Design review of the part built by this model. Coordinates are the model's own, in mm. Face numbers are marked on the shaded views. A direction names the side the tool comes from. Give positions to 0.01 mm unless a question says otherwise; leave off trailing zeros. Write each loop counter-clockwise with the first axis right and the second up, starting at its lowest first coordinate (ties: lowest second). Pieces come first, ordered by that corner, then holes. Notation, with made-up numbers: (83.25, 58.5) -> (107.25, 58.5) arc R30 cw to (107.25, 96.5) -> close; hole circle Ø6 at (-0.5, 8.25). An arc over 180 degrees is marked (long way). Use CSV: the item, a comma, the result in double quotes.
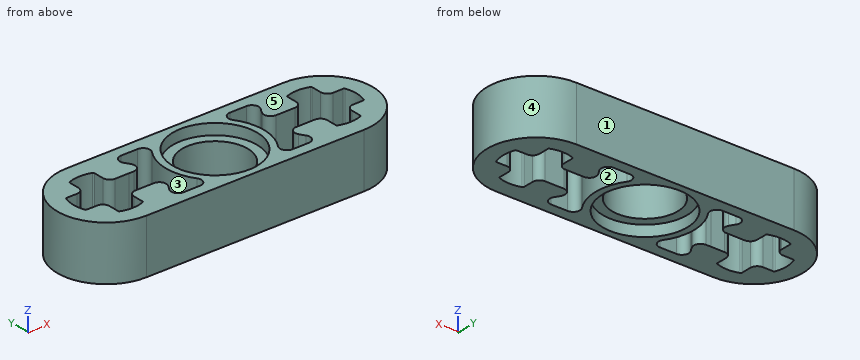
Solid Edge part; units mm, degrees
sketch "Sketch1" plane through (0, 0, 0) normal (0, 0, 1) x (1, 0, 0)
  line L0 (0, 0) -> (0, 3.6)
  line L1 (0, 3.6) -> (8, 3.6)
  line L2 (8, -3.6) -> (0, -3.6)
  line L3 (0, -3.6) -> (0, 0)
  arc A0 (8, 3.6) -> (8, -3.6) centre (8, 0) cw
extrude "ExtrudedProtrusion_1" add sketch "Sketch1" along normal blind 4
mirror "Mirror1" about plane through (0, 0, 0) normal (-1, 0, 0) of "ExtrudedProtrusion_1"
sketch "Sketch2" plane through (0, 0, 0) normal (0, -1, 0) x (1, 0, 0)
  line L0 (0, 0) -> (0, 4)
  line L1 (0, 4) -> (3.1, 4)
  line L2 (3.1, 4) -> (3.1, 3.2)
  line L3 (3.1, 3.2) -> (2.4, 3.2)
  line L4 (2.4, 3.2) -> (2.4, 0.8)
  line L5 (2.4, 0.8) -> (3.1, 0.8)
  line L6 (3.1, 0.8) -> (3.1, 0)
  line L7 (3.1, 0) -> (0, 0)
revolve "RevolvedCutout1" cut sketch "Sketch2" angle 360 about axis through (0, 0, 54) along (0, 0, -1)
sketch "Sketch3" plane through (0, 0, 4) normal (0, 0, 1) x (1, 0, 0)
  line L0 (-5.7373, 2.8) -> (-2.2627, 2.8)
  line L1 (-5.7373, -2.8) -> (-2.2627, -2.8)
  arc A0 (-4.5143, -0.9) -> (-5.7373, -2.8) centre (-8, 0) cw
  line L2 (-5.6, -0.9) -> (-4.5143, -0.9)
  line L3 (-7.0981, -0.9) -> (-5.6, -0.9)
  line L4 (-7.0981, -0.9) -> (-7.0981, -2.2241)
  arc A1 (-7.0981, -2.2241) -> (-8.8981, -2.2256) centre (-8, 0) cw
  line L5 (-8.8981, -2.2256) -> (-8.8981, -0.9)
  line L6 (-10.2249, -0.9) -> (-8.8981, -0.9)
  arc A2 (-10.2249, -0.9) -> (-10.2249, 0.9) centre (-8, 0) cw
  line L7 (-8.8981, 0.9) -> (-10.2249, 0.9)
  line L8 (-8.8981, 0.9) -> (-8.8981, 2.2256)
  line L9 (-7.0981, 2.2241) -> (-7.0981, 0.9)
  line L10 (-5.6, 0.9) -> (-7.0981, 0.9)
  line L11 (-5.6, 0.9) -> (-4.5143, 0.9)
  arc A3 (-4.5143, 0.9) -> (-5.7373, 2.8) centre (-8, 0) ccw
  arc A4 (-8.8981, 2.2256) -> (-7.0981, 2.2241) centre (-8, 0) cw
  arc A5 (-2.2627, 2.8) -> (-2.2627, -2.8) centre (0, 0) ccw
  line L12 (2.2627, -2.8) -> (5.7373, -2.8)
  arc A6 (5.7373, -2.8) -> (4.5143, -0.9) centre (8, 0) cw
  line L13 (7.111, -0.9) -> (4.5143, -0.9)
  line L14 (7.111, -2.2293) -> (7.111, -0.9)
  arc A7 (8.911, -2.2204) -> (7.111, -2.2293) centre (8, 0) cw
  line L15 (8.911, -0.9) -> (8.911, -2.2204)
  line L16 (10.2249, -0.9) -> (8.911, -0.9)
  arc A8 (10.2249, 0.9) -> (10.2249, -0.9) centre (8, 0) cw
  line L17 (10.2249, 0.9) -> (8.911, 0.9)
  line L18 (8.911, 2.2204) -> (8.911, 0.9)
  line L19 (7.111, 0.9) -> (7.111, 2.2293)
  line L20 (7.111, 0.9) -> (4.5143, 0.9)
  line L21 (2.2627, 2.8) -> (5.7373, 2.8)
  arc A9 (2.2627, 2.8) -> (2.2627, -2.8) centre (0, 0) cw
  arc A10 (5.7373, 2.8) -> (4.5143, 0.9) centre (8, 0) ccw
  arc A11 (7.111, 2.2293) -> (8.911, 2.2204) centre (8, 0) cw
  dimension "D1" = 2.2627
extrude "ExtrudedCutout_1" cut sketch "Sketch3" against normal blind 30
fillet "Round_1" radius 0.5 20 edges at (-5.7373, 2.8, 2) (-2.2627, 2.8, 2) (5.7373, 2.8, 2) (-7.0981, 0.9, 2) (-8.8981, 0.9, 2) (-8.8981, -0.9, 2) (-7.0981, -0.9, 2) (-4.5143, -0.9, 2) (-4.5143, 0.9, 2) (-2.2627, -2.8, 2) (-5.7373, -2.8, 2) (7.111, -0.9, 2) (7.111, 0.9, 2) (8.911, 0.9, 2) (8.911, -0.9, 2) (4.5143, 0.9, 2) (4.5143, -0.9, 2) (2.2627, -2.8, 2) (5.7373, -2.8, 2) (2.2627, 2.8, 2)
fillet "Round_2" radius 0.1 12 edges at (-8.8981, 2.2256, 2) (-7.0981, 2.2241, 2) (-10.2249, 0.9, 2) (-10.2249, -0.9, 2) (-8.8981, -2.2256, 2) (-7.0981, -2.2241, 2) (8.911, -2.2204, 2) (10.2249, -0.9, 2) (10.2249, 0.9, 2) (8.911, 2.2204, 2) (7.111, -2.2293, 2) (7.111, 2.2293, 2)
(1) Clearance check with flat-ended pins moving along their axes: pin 1 (0.6 mm diameter, centred on y = 1.5, z = 2, fed in from +X); pin 2 (0.6 mm diameter, centred on y = 2, z = 2, fed in from -X); pin 3 (3.5 mm diameter, centred on x = 0, y = 0, fed in from +Z); pin 4 (1 mm diameter, centred on x = -0.5, y = 2.5, fed in from +Z). State where each tip first meets the part, or that it passes through.
Established:
pin 1,"stops at x = 11.39"
pin 2,"stops at x = -11.17"
pin 3,"passes through"
pin 4,"stops at z = 3.2"
(2) Take a section at A-A (x = 0). Write out the cut boundary in (y, z).
Established:
outline,"(-3.6, 0) -> (-3.1, 0) -> (-3.1, 0.8) -> (-2.4, 0.8) -> (-2.4, 3.2) -> (-3.1, 3.2) -> (-3.1, 4) -> (-3.6, 4) -> close; (2.4, 0.8) -> (3.1, 0.8) -> (3.1, 0) -> (3.6, 0) -> (3.6, 4) -> (3.1, 4) -> (3.1, 3.2) -> (2.4, 3.2) -> close"
(3) Take a section at B-B (y = 0). Write out the cut boundary in (x, z).
Established:
outline,"(-11.6, 0) -> (-10.4, 0) -> (-10.4, 4) -> (-11.6, 4) -> close; (-3.6, 0) -> (-3.1, 0) -> (-3.1, 0.8) -> (-2.4, 0.8) -> (-2.4, 3.2) -> (-3.1, 3.2) -> (-3.1, 4) -> (-3.6, 4) -> close; (2.4, 0.8) -> (3.1, 0.8) -> (3.1, 0) -> (3.6, 0) -> (3.6, 4) -> (3.1, 4) -> (3.1, 3.2) -> (2.4, 3.2) -> close; (10.4, 0) -> (11.6, 0) -> (11.6, 4) -> (10.4, 4) -> close"
(4) Tool access review of the marked faces 1 and 2: name each direction out of +Z, -Z, +X, -X, +Y, -Y from which nothing blocks a thin tool from reaching the whole face with its end or side.
Established:
face 1,"+Z, -Z, +X, -X, +Y"
face 2,"+Z, -Z"
(5) Take a section at C-C (z = 2.65). State how many separate pieces and enclosed holes the cut face has, then the cut area to 3 significant figures.
Established:
separate pieces,"1"
enclosed holes,"3"
area,"89.2 mm2"
(6) Take a section at D-D (x = 8.5). Write out the cut boundary in (y, z).
Established:
outline,"(-3.57, 0) -> (-2.35, 0) -> (-2.35, 4) -> (-3.57, 4) -> close; (2.35, 0) -> (3.57, 0) -> (3.57, 4) -> (2.35, 4) -> close"
(7) For line 1 along X through (y, z) = (0, 1.45); line 2 along Y through (x, z) = (0, 0.6); line 3 along X through (y, z) = (0, 3.6), list the stretches that pass through material, from the lowest coordinate up. Write a range as [from, to].
Established:
line 1,"x = [-11.6, -10.4], [-3.6, -2.4], [2.4, 3.6], [10.4, 11.6]"
line 2,"y = [-3.6, -3.1], [3.1, 3.6]"
line 3,"x = [-11.6, -10.4], [-3.6, -3.1], [3.1, 3.6], [10.4, 11.6]"
(8) Mouldability with a two-part tool opening along X and no side actions: class the marked faces 3, 4 and 5 as +X half, -X half, draft (parallel to the pull), parting line (faces both ways), or undercut.
Established:
face 3,"undercut"
face 4,"+X half"
face 5,"draft"
